Source: CAD feature listing. Evaluate the final solid. Frame: model axes, mm. A direction names the side the tool comes from. Give positions to 0.01 mm unless a question says otherwise; leave off trailing zeros. Order: outer loops, then holes, each group sorted by start corner. A loop starts at its lowest first (then second) coordinate and runs counter-clockwise, first axis right, second up.
from build123d import *

# Parameters (mm, degrees)
BASE_FLANGE1_DEPTH = 490.75


# Sheet-metal steps are written as plain solids
with BuildPart() as part:
    # Sketch1 → Base-Flange1 (new, symmetric)
    with BuildSketch(Plane(origin=(0, 0, 0), x_dir=(1, 0, 0), z_dir=(0, 1, 0))):
        with BuildLine():
            Line((9.5, 59.25), (9.5, 68.0134))
            ThreePointArc((9.5, 68.0134), (10.081861668, 69.418138332), (11.4866, 70))
            Line((11.4866, 70), (37.5134, 70))
            ThreePointArc((37.5134, 70), (38.918138332, 69.418138332), (39.5, 68.0134))
            Line((39.5, 68.0134), (39.5, 23))
            Line((39.5, 23), (39.5, 8.562771629))
            ThreePointArc((39.5, 8.562771629), (39.724914644, 8.032905932), (40.262306969, 7.826620346))
            Line((40.262306969, 7.826620346), (42.153527557, 7.892663224))
            ThreePointArc((42.153527557, 7.892663224), (42.675221066, 8.135932903), (42.862626267, 8.680197126))
            Line((42.862626267, 8.680197126), (42.359529101, 15.874821789))
            ThreePointArc((42.359529101, 15.874821789), (42.88838258, 17.368257942), (44.341289843, 18))
            Line((44.341289843, 18), (52.2634, 18))
            ThreePointArc((52.2634, 18), (53.668138332, 17.418138332), (54.25, 16.0134))
            Line((54.25, 16.0134), (54.25, -21.0134))
            ThreePointArc((54.25, -21.0134), (53.668138332, -22.418138332), (52.2634, -23))
            Line((52.2634, -23), (40.2366, -23))
            ThreePointArc((40.2366, -23), (39.715745145, -23.215745145), (39.5, -23.7366))
            Line((39.5, -23.7366), (39.5, -68.0134))
            ThreePointArc((39.5, -68.0134), (38.918138332, -69.418138332), (37.5134, -70))
            Line((37.5134, -70), (11.4866, -70))
            ThreePointArc((11.4866, -70), (10.081861668, -69.418138332), (9.5, -68.0134))
            Line((9.5, -68.0134), (9.5, -59.25))
            Line((9.5, -59.25), (10.75, -59.25))
            Line((10.75, -59.25), (10.75, -68.0134))
            ThreePointArc((10.75, -68.0134), (10.965745145, -68.534254855), (11.4866, -68.75))
            Line((11.4866, -68.75), (37.5134, -68.75))
            ThreePointArc((37.5134, -68.75), (38.034254855, -68.534254855), (38.25, -68.0134))
            Line((38.25, -68.0134), (38.25, -23.7366))
            ThreePointArc((38.25, -23.7366), (38.831861668, -22.331861668), (40.2366, -21.75))
            Line((40.2366, -21.75), (52.2634, -21.75))
            ThreePointArc((52.2634, -21.75), (52.784254855, -21.534254855), (53, -21.0134))
            Line((53, -21.0134), (53, 16.0134))
            ThreePointArc((53, 16.0134), (52.784254855, 16.534254855), (52.2634, 16.75))
            Line((52.2634, 16.75), (44.341289843, 16.75))
            ThreePointArc((44.341289843, 16.75), (43.802574707, 16.515759992), (43.606484164, 15.962017381))
            Line((43.606484164, 15.962017381), (44.10958133, 8.767392718))
            ThreePointArc((44.10958133, 8.767392718), (43.604152098, 7.299519645), (42.197151928, 6.64342469))
            Line((42.197151928, 6.64342469), (40.30593134, 6.577381812))
            ThreePointArc((40.30593134, 6.577381812), (38.856591681, 7.133731182), (38.25, 8.562771629))
            Line((38.25, 8.562771629), (38.25, 23))
            Line((38.25, 23), (38.25, 68.0134))
            ThreePointArc((38.25, 68.0134), (38.034254855, 68.534254855), (37.5134, 68.75))
            Line((37.5134, 68.75), (11.4866, 68.75))
            ThreePointArc((11.4866, 68.75), (10.965745145, 68.534254855), (10.75, 68.0134))
            Line((10.75, 68.0134), (10.75, 59.25))
            Line((10.75, 59.25), (9.5, 59.25))
        make_face()
    extrude(amount=BASE_FLANGE1_DEPTH, both=True)


solid = part.part
(1) Line query: line 1 along X through (y, z) = (125, -61); line 2 along Z through (x, y) = (21, -418); line 3 along Z through (x, y) = (51, 216.5). Output: solid intervals per line, ascending.
(2) Draft query along X for faces 1 (the flat face through (38.25, 7, 46)), 2 (the flat face through (24, 7, 68.75)), 3 (the flat face through (54.25, 7, 2)), 4 (the flat face through (24, 7, -70)). Return one class per face: +X half, -X half, draft (parallel to the pull), parting line (faces both ways), or undercut.
(3) Section A-A, the plane x = 27. Return loops of the section in (y, z), plus the area to 3 significant figures.
(4) Access query for faces 5 (the flat face through (39.5, 7, 46)), 6 (the flat face through (39, -490.75, -11)), 7 (the flat face through (25, 7, -68.75)). Directions: +Z, -Z, +X, -X, +Y, -Y. A direction counts if a zero-diameter tool reaches every point of the face in a straight line with its end or side. Return the directions, or none.
(5) Section B-B, the plane z = -50. Return loops of the section in (x, y), plus the area to 3 significant figures.
(6) Pin query (flat end, axial travel): pin 1 Ø5 at (x, y) = (40.5, -212) entering from +Z; pin 2 Ø7 at (y, z) = (-153, -63) entering from +X; pin 3 Ø3 at (y, z) = (111.5, -43.5) entering from -X. Return the tip coordinate at first contact, or that it passes through.
Checks:
1. line 1: x = 9.5 to 10.75, 38.25 to 39.5
1. line 2: z = -70 to -68.75, 68.75 to 70
1. line 3: z = -18 to -16.75, 21.75 to 23
2. face 1: undercut
2. face 2: undercut
2. face 3: +X half
2. face 4: draft
3. outline: (-490.75, -70) - (490.75, -70) - (490.75, -68.75) - (-490.75, -68.75) - close; (-490.75, 68.75) - (490.75, 68.75) - (490.75, 70) - (-490.75, 70) - close
3. area: 2,450 mm2
4. face 5: +Z, +X, +Y, -Y
4. face 6: +Z, -Z, +X, -X, -Y
4. face 7: +Y, -Y
5. outline: (38.25, -490.75) - (39.5, -490.75) - (39.5, 490.75) - (38.25, 490.75) - close
5. area: 1,230 mm2
6. pin 1: stops at z = 69.94
6. pin 2: stops at x = 39.5
6. pin 3: stops at x = 38.25
